from build123d import *

# Parameters (mm, degrees)
BOSS_EXTRUDE1_DEPTH           = 12.7
SKETCH2_R                     = 63.5
CUT_EXTRUDE2_DEPTH            = 12.7
CUT_EXTRUDE3_DEPTH            = 1.27
SKETCH4_R                     = 2.4003
CUT_EXTRUDE4_DEPTH            = 2.27
CUT_EXTRUDE4_DEPTH_BACK       = 12.43
CBORE_FOR_M6_SHCS2_AT_2_COUNT = 2
CBORE_FOR_M6_SHCS2_AT_2_PITCH = 139.7
CBORE_FOR_M6_SHCS2_AT_3_COUNT = 2
CBORE_FOR_M6_SHCS2_AT_3_PITCH = 139.7
CBORE_FOR_M6_SHCS2_AT_4_COUNT = 2
CBORE_FOR_M6_SHCS2_AT_4_PITCH = 139.7
CBORE_FOR_M6_SHCS2_AT_5_COUNT = 2
CBORE_FOR_M6_SHCS2_AT_5_PITCH = 139.7
CBORE_FOR_M6_SHCS2_AT_6_COUNT = 2
CBORE_FOR_M6_SHCS2_AT_6_PITCH = 139.7
CBORE_FOR_M6_SHCS2_AT_7_COUNT = 2
CBORE_FOR_M6_SHCS2_AT_7_PITCH = 139.7
SKETCH7_R                     = 25.4
BOSS_EXTRUDE2_DEPTH           = 11.43
SKETCH8_R                     = 18.542
CUT_EXTRUDE5_DEPTH            = 6.35
CBORE_FOR_M3_SHCS1_AT_2_COUNT = 2
CBORE_FOR_M3_SHCS1_AT_2_PITCH = 15.499969
CBORE_FOR_M3_SHCS1_AT_3_COUNT = 2
CBORE_FOR_M3_SHCS1_AT_3_PITCH = 26.846733824
CBORE_FOR_M3_SHCS1_AT_4_COUNT = 2
CBORE_FOR_M3_SHCS1_AT_4_PITCH = 30.999938
CBORE_FOR_M3_SHCS1_AT_5_COUNT = 2
CBORE_FOR_M3_SHCS1_AT_5_PITCH = 26.846733824
CBORE_FOR_M3_SHCS1_AT_6_COUNT = 2
CBORE_FOR_M3_SHCS1_AT_6_PITCH = 15.499969
SKETCH11_R                    = 6.223
CUT_EXTRUDE6_DEPTH            = 11.43


with BuildPart() as part:
    # Sketch1 → Boss-Extrude1 (new body)
    with BuildSketch(Plane(origin=(0, 0, 0), x_dir=(1, 0, 0), z_dir=(0, 1, 0))):
        with BuildLine():
            Line((-25.4, 123.785916909), (-25.4, 150.268426491))
            ThreePointArc((-25.4, 150.268426491), (0, 152.4), (25.4, 150.268426491))
            Line((25.4, 150.268426491), (25.4, 123.785916909))
            ThreePointArc((25.4, 123.785916909), (63.1825, 109.435300149), (94.501748674, 83.890003711))
            Line((94.501748674, 83.890003711), (117.436274728, 97.131258501))
            ThreePointArc((117.436274728, 97.131258501), (131.982271537, 76.2), (142.836274728, 53.137167989))
            Line((142.836274728, 53.137167989), (119.901748674, 39.895913198))
            ThreePointArc((119.901748674, 39.895913198), (126.365, 0), (119.901748674, -39.895913198))
            Line((119.901748674, -39.895913198), (142.836274728, -53.137167989))
            ThreePointArc((142.836274728, -53.137167989), (131.982271537, -76.2), (117.436274728, -97.131258501))
            Line((117.436274728, -97.131258501), (94.501748674, -83.890003711))
            ThreePointArc((94.501748674, -83.890003711), (63.1825, -109.435300149), (25.4, -123.785916909))
            Line((25.4, -123.785916909), (25.4, -150.268426491))
            ThreePointArc((25.4, -150.268426491), (0, -152.4), (-25.4, -150.268426491))
            Line((-25.4, -150.268426491), (-25.4, -123.785916909))
            ThreePointArc((-25.4, -123.785916909), (-63.1825, -109.435300149), (-94.501748674, -83.890003711))
            Line((-94.501748674, -83.890003711), (-117.436274728, -97.131258501))
            ThreePointArc((-117.436274728, -97.131258501), (-131.982271537, -76.2), (-142.836274728, -53.137167989))
            Line((-142.836274728, -53.137167989), (-119.901748674, -39.895913198))
            ThreePointArc((-119.901748674, -39.895913198), (-126.365, 0), (-119.901748674, 39.895913198))
            Line((-119.901748674, 39.895913198), (-142.836274728, 53.137167989))
            ThreePointArc((-142.836274728, 53.137167989), (-131.982271537, 76.2), (-117.436274728, 97.131258501))
            Line((-117.436274728, 97.131258501), (-94.501748674, 83.890003711))
            ThreePointArc((-94.501748674, 83.890003711), (-63.1825, 109.435300149), (-25.4, 123.785916909))
        make_face()
    extrude(amount=BOSS_EXTRUDE1_DEPTH)

    # Sketch2 → Cut-Extrude2 (cut)
    with BuildSketch(Plane(origin=(0, 0, 0), x_dir=(1, 0, 0), z_dir=(0, 1, 0))):
        Circle(SKETCH2_R)
    extrude(amount=CUT_EXTRUDE2_DEPTH, mode=Mode.SUBTRACT)

    # Sketch3 → Cut-Extrude3 (cut)
    with BuildSketch(Plane(origin=(0, 12.7, 0), x_dir=(1, 0, 0), z_dir=(0, 1, 0))):
        with BuildLine():
            Line((-76.2, 16.800520825), (-76.2, 76.2))
            Line((-76.2, 76.2), (76.2, 76.2))
            Line((76.2, 76.2), (76.2, -76.2))
            Line((76.2, -76.2), (-76.2, -76.2))
            Line((-76.2, -76.2), (-76.2, -16.800520825))
            ThreePointArc((-76.2, -16.800520825), (-82.55, 0), (-76.2, 16.800520825))
        make_face()
    extrude(amount=-CUT_EXTRUDE3_DEPTH, mode=Mode.SUBTRACT)

    # Sketch4 → Cut-Extrude4 (cut, two sides)
    with BuildSketch(Plane(origin=(0, 11.43, 0), x_dir=(1, 0, 0), z_dir=(0, 1, 0))) as cut_extrude4_sk:
        with Locations((-60.5282, 60.5282)):
            Circle(SKETCH4_R)
        with Locations((-60.5282, -60.5282)):
            Circle(SKETCH4_R)
        with Locations((60.5282, -60.5282)):
            Circle(SKETCH4_R)
        with Locations((60.5282, 60.5282)):
            Circle(SKETCH4_R)
    extrude(amount=CUT_EXTRUDE4_DEPTH, mode=Mode.SUBTRACT)
    extrude(cut_extrude4_sk.sketch, amount=-CUT_EXTRUDE4_DEPTH_BACK, mode=Mode.SUBTRACT)

    # Sketch6 → CBORE for M6 SHCS2 (revolve, cut)
    with BuildSketch(Plane(origin=(0, 12.7, 0), x_dir=(0, 0, 1), z_dir=(1, 0, 0))):
        Polygon((0, 0), (0, 12.7), (3.3, 12.7), (3.3, 6), (5.5, 6), (5.5, 0.025), (5.525, 0), align=None)
    cbore_for_m6_shcs2 = revolve(axis=Axis((0, 19.05, 0), (0, -1, 0)), mode=Mode.SUBTRACT)

    # CBORE for M6 SHCS2 at 2: CBORE for M6 SHCS2 ×2
    with Locations(*[(0, 0, -i * CBORE_FOR_M6_SHCS2_AT_2_PITCH) for i in range(1, CBORE_FOR_M6_SHCS2_AT_2_COUNT)]):
        add(cbore_for_m6_shcs2, mode=Mode.SUBTRACT)

    # CBORE for M6 SHCS2 at 3: CBORE for M6 SHCS2 ×2
    with Locations(*[Vector(0.866025404, 0, -0.5) * (i * CBORE_FOR_M6_SHCS2_AT_3_PITCH) for i in range(1, CBORE_FOR_M6_SHCS2_AT_3_COUNT)]):
        add(cbore_for_m6_shcs2, mode=Mode.SUBTRACT)

    # CBORE for M6 SHCS2 at 4: CBORE for M6 SHCS2 ×2
    with Locations(*[Vector(0.866025404, 0, 0.5) * (i * CBORE_FOR_M6_SHCS2_AT_4_PITCH) for i in range(1, CBORE_FOR_M6_SHCS2_AT_4_COUNT)]):
        add(cbore_for_m6_shcs2, mode=Mode.SUBTRACT)

    # CBORE for M6 SHCS2 at 5: CBORE for M6 SHCS2 ×2
    with Locations(*[(0, 0, i * CBORE_FOR_M6_SHCS2_AT_5_PITCH) for i in range(1, CBORE_FOR_M6_SHCS2_AT_5_COUNT)]):
        add(cbore_for_m6_shcs2, mode=Mode.SUBTRACT)

    # CBORE for M6 SHCS2 at 6: CBORE for M6 SHCS2 ×2
    with Locations(*[Vector(-0.866025404, 0, 0.5) * (i * CBORE_FOR_M6_SHCS2_AT_6_PITCH) for i in range(1, CBORE_FOR_M6_SHCS2_AT_6_COUNT)]):
        add(cbore_for_m6_shcs2, mode=Mode.SUBTRACT)

    # CBORE for M6 SHCS2 at 7: CBORE for M6 SHCS2 ×2
    with Locations(*[Vector(-0.866025404, 0, -0.5) * (i * CBORE_FOR_M6_SHCS2_AT_7_PITCH) for i in range(1, CBORE_FOR_M6_SHCS2_AT_7_COUNT)]):
        add(cbore_for_m6_shcs2, mode=Mode.SUBTRACT)

    # Sketch7 → Boss-Extrude2 (add)
    with BuildSketch(Plane.XZ):
        with Locations((-57.15, 0)):
            Circle(SKETCH7_R)
    extrude(amount=-BOSS_EXTRUDE2_DEPTH)

    # Sketch8 → Cut-Extrude5 (cut)
    with BuildSketch(Plane(origin=(0, 0, 0), x_dir=(-1, 0, 0), z_dir=(0, -1, 0))):
        with Locations((57.15, 0)):
            Circle(SKETCH8_R)
    extrude(amount=-CUT_EXTRUDE5_DEPTH, mode=Mode.SUBTRACT)

    # Sketch10 → CBORE for M3 SHCS1 (revolve, cut)
    with BuildSketch(Plane(origin=(-70.573366912, 11.43, 7.7499845), x_dir=(0, 0, 1), z_dir=(1, 0, 0))):
        Polygon((0, 0), (0, 6.101463052), (1.7, 5.08), (1.7, 3), (3.25, 3), (3.25, 0.025), (3.275, 0), align=None)
    cbore_for_m3_shcs1 = revolve(axis=Axis((-70.573366912, 17.78, 7.7499845), (0, -1, 0)), mode=Mode.SUBTRACT)

    # CBORE for M3 SHCS1 at 2: CBORE for M3 SHCS1 ×2
    with Locations(*[Vector(0.866025404, 0, 0.5) * (i * CBORE_FOR_M3_SHCS1_AT_2_PITCH) for i in range(1, CBORE_FOR_M3_SHCS1_AT_2_COUNT)]):
        add(cbore_for_m3_shcs1, mode=Mode.SUBTRACT)

    # CBORE for M3 SHCS1 at 3: CBORE for M3 SHCS1 ×2
    with Locations(*[(i * CBORE_FOR_M3_SHCS1_AT_3_PITCH, 0, 0) for i in range(1, CBORE_FOR_M3_SHCS1_AT_3_COUNT)]):
        add(cbore_for_m3_shcs1, mode=Mode.SUBTRACT)

    # CBORE for M3 SHCS1 at 4: CBORE for M3 SHCS1 ×2
    with Locations(*[Vector(0.866025404, 0, -0.5) * (i * CBORE_FOR_M3_SHCS1_AT_4_PITCH) for i in range(1, CBORE_FOR_M3_SHCS1_AT_4_COUNT)]):
        add(cbore_for_m3_shcs1, mode=Mode.SUBTRACT)

    # CBORE for M3 SHCS1 at 5: CBORE for M3 SHCS1 ×2
    with Locations(*[Vector(0.5, 0, -0.866025404) * (i * CBORE_FOR_M3_SHCS1_AT_5_PITCH) for i in range(1, CBORE_FOR_M3_SHCS1_AT_5_COUNT)]):
        add(cbore_for_m3_shcs1, mode=Mode.SUBTRACT)

    # CBORE for M3 SHCS1 at 6: CBORE for M3 SHCS1 ×2
    with Locations(*[(0, 0, -i * CBORE_FOR_M3_SHCS1_AT_6_PITCH) for i in range(1, CBORE_FOR_M3_SHCS1_AT_6_COUNT)]):
        add(cbore_for_m3_shcs1, mode=Mode.SUBTRACT)

    # Sketch11 → Cut-Extrude6 (cut)
    with BuildSketch(Plane.XZ):
        with Locations((-50.1500013, 0)):
            Circle(SKETCH11_R)
    extrude(amount=-CUT_EXTRUDE6_DEPTH, mode=Mode.SUBTRACT)


solid = part.part
Verification items for the finished model (mm, model axes). A direction names the side the tool comes from. Give positions to 0.01 mm unless a question says otherwise; leave off trailing zeros. Loops run counter-clockwise (first coordinate to the right, second up) from the corner with the lowest first, then second, coordinate; pieces in that order, holes last. Notation, with made-up numbers: (75, 64.5) - (97, 64.5) arc R12 cw to (97, 74.5) - close; hole circle Ø10 at (-27, 54.5). An arc over 180 degrees is marked (long way). Write each question's results on one line, items separated by ' | '.
1) Material ranges on L1, parallel to X at y = 7.5, z = -71.5; L2, parallel to X at y = 5.25, z = -89.5; L3, parallel to Z at x = -27.5, y = 10.5, recorded low to high. Write a range as from..to.
Solution:
L1: -134.59..-126.23, -115.74..115.74, 126.23..134.59 | L2: -123.35..-104.22, -89.21..89.21, 104.22..123.35 | L3: -123.34..-57.24, 57.24..123.34
2) Mould release check, pull along Z, two halves, no side actions. Record for faces 4 (the cylindrical face through (-73.796, 9.938, 7.327)), 5 (the flat face through (106.13, 6.261, 90.603)), 6 (the flat face through (25.4, 6, 137)), 7 (the cylindrical face through (123.911, 3.397, 71.373)): pulls with the +Z half, pulls with the -Z half, needs draft (parallel to the pull), parting line crosses it, or undercut.
Solution:
face 4: undercut | face 5: pulls with the +Z half | face 6: needs draft | face 7: undercut
3) Depth check by flat-ended pin: P1, Ø5, axis at x = -43.5, z = -6.5, coming from the +Y side; P2, Ø1, axis at y = 11, z = -74.5, coming from the -X side; P3, Ø11, axis at x = -61, z = -0.5, coming from the -Y side. Enter the tip coordinate at first touch or a pass-through.
Solution:
P1: y = 11.43 | P2: x = -133.23 | P3: y = 6.35
4) Tool access check on faces 1 (the flat face through (-131.53, 6.26, 46.61)), 2 (the cylindrical face through (-62.69, 6.26, 109.72)), 3 (the cylindrical face through (-82.55, 12.07, 0.26)). Record the directions out of +Z, -Z, +X, -X, +Y, -Y that give a thin tool (end or side, any length) a straight path to the whole face; none if there is none.
Solution:
face 1: -X, +Y, -Y | face 2: +Z, +Y, -Y | face 3: +Y
5) Sectioned sample at C-C on z = -45.5. Record the boundary of the cut face in (x, y).
Solution:
outline: (-129.61, 0) - (-44.29, 0) - (-44.29, 11.43) - (-76.2, 11.43) - (-76.2, 12.7) - (-129.61, 12.7) - close; (44.29, 0) - (129.61, 0) - (129.61, 12.7) - (76.2, 12.7) - (76.2, 11.43) - (44.29, 11.43) - close
6) Sectioned sample at B-B on x = 33. Record the boundary of the cut face in (y, z).
Solution:
outline: (0, -121.98) - (12.7, -121.98) - (12.7, -76.2) - (11.43, -76.2) - (11.43, -54.25) - (0, -54.25) - close; (0, 54.25) - (11.43, 54.25) - (11.43, 76.2) - (12.7, 76.2) - (12.7, 121.98) - (0, 121.98) - close
7) Sectioned sample at D-D on x = -50.5. Record the boundary of the cut face in (y, z).
Solution:
outline: (0, -115.84) - (12.7, -115.84) - (12.7, -76.2) - (11.43, -76.2) - (11.43, -38.5) - (0, -38.5) - close; (0, -24.51) - (11.43, -24.51) - (11.43, -6.21) - (6.35, -6.21) - (6.35, -17.31) - (0, -17.31) - close; (0, 17.31) - (6.35, 17.31) - (6.35, 6.21) - (11.43, 6.21) - (11.43, 24.51) - (0, 24.51) - close; (0, 38.5) - (11.43, 38.5) - (11.43, 76.2) - (12.7, 76.2) - (12.7, 115.84) - (0, 115.84) - close
8) Sectioned sample at A-A on z = 0. Record the boundary of the cut face in (x, y) (3 decimals).
Solution:
outline: (-126.365, 0) - (-75.692, 0) - (-75.692, 6.35) - (-56.373, 6.35) - (-56.373, 11.43) - (-82.55, 11.43) - (-82.55, 12.7) - (-126.365, 12.7) - close; (-43.927, 6.35) - (-38.608, 6.35) - (-38.608, 0) - (-31.75, 0) - (-31.75, 11.43) - (-43.927, 11.43) - close; (63.5, 0) - (126.365, 0) - (126.365, 12.7) - (76.2, 12.7) - (76.2, 11.43) - (63.5, 11.43) - close
